Part print with two shaded views. Sizes in mm from the minimum x, y, z corner. Give positions to 0.01 mm unless a question says otherwise; leave off trailing zeros. Write each loop counter-clockwise with the first axis right and the second up, starting at its lowest first coordinate (ties: lowest second). Pieces come first, ordered by that corner, then holes.
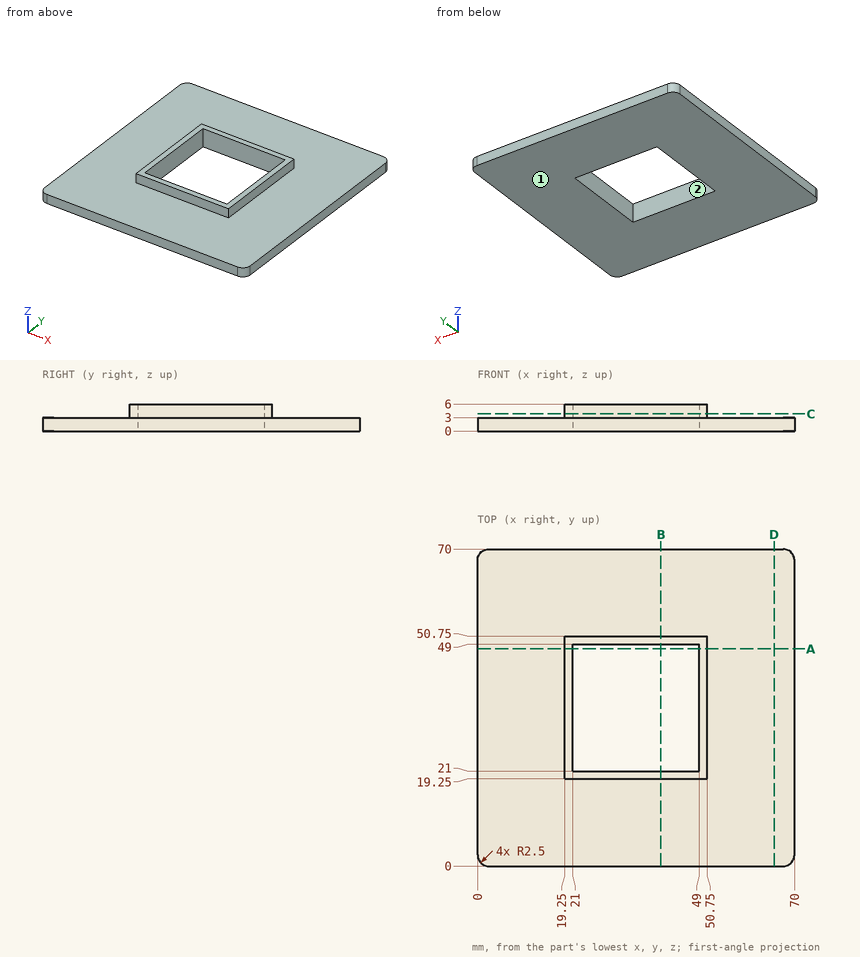
1) Saw through at D-D, the plane x = 65.5. Write the cut outline in (y, z).
Answers follow:
outline: (0, 0) - (70, 0) - (70, 3) - (0, 3) - close
2) Saw through at C-C, the plane z = 3.8. Write the cut outline in (x, y).
Answers follow:
outline: (19.25, 19.25) - (50.75, 19.25) - (50.75, 50.75) - (19.25, 50.75) - close; hole (21, 21) - (49, 21) - (49, 49) - (21, 49) - close
3) Two-plate mould, pull along Y, no slides. Class the marked faces 1 and 2: +Y half, -Y half, draft (parallel to the pull), parting line (faces both ways), or undercut.
Answers follow:
face 1: draft
face 2: undercut
4) Wall check: L1, parallel to X at y = 41, z = 1.95; L2, parallel to X at y = 34, z = 3.45. Give the ranges that are in metal, low to high.
Answers follow:
L1: x = 0 to 21, 49 to 70
L2: x = 19.25 to 21, 49 to 50.75
5) Saw through at A-A, the plane y = 48. Write the cut outline in (x, z), then the cut area to 4 significant figures.
Answers follow:
outline: (0, 0) - (21, 0) - (21, 6) - (19.25, 6) - (19.25, 3) - (0, 3) - close; (49, 0) - (70, 0) - (70, 3) - (50.75, 3) - (50.75, 6) - (49, 6) - close
area: 136.5 mm2
6) Pin check, flat tips, straight feed: pin 1 Ø1.5 at (x, z) = (29.5, 5) entering from +Y; pin 2 Ø2.5 at (y, z) = (31, 5) entering from -X; pin 3 Ø2 at (x, y) = (35.5, 16.5) entering from +Z. Stop position of each tip, or through.
Answers follow:
pin 1: stops at y = 50.75
pin 2: stops at x = 19.25
pin 3: stops at z = 3
